from build123d import *

# Parameters (mm, degrees)
F0_R        = 15.113
F0_R_2      = 2.0114491118
F1_DEPTH    = 2.54
F2_T1_DEPTH = 2.54
F2_T3_DEPTH = 27.94


# Not quite as in the source:
# - a fillet or chamfer that OpenCascade refuses, or shapes differently, is made with other operations: its cross-section is extruded or revolved along the edge and cut away or added


with BuildPart() as f1:
    # F0 (on Top) → F1 (new body)
    with BuildSketch(Plane.XY):
        with BuildLine():
            Line((27.3455847055, 4.693207435), (17.2810431679, 4.693207435))
            ThreePointArc((17.2810431679, 4.693207435), (-17.907, 0), (17.2810431679, -4.693207435))
            Line((17.2810431679, -4.693207435), (27.3455847055, -4.693207435))
            Line((27.3455847055, -4.693207435), (27.3455847055, 4.693207435))
        make_face()
        Circle(F0_R, mode=Mode.SUBTRACT)
        with Locations((22.3272647709, 0)):
            Circle(F0_R_2, mode=Mode.SUBTRACT)
    extrude(amount=F1_DEPTH)

    # F2: fillet of radius 5.08 on 4 edges, made by hand

    # F2_s2 → F2_t1 (join)
    with BuildSketch(Plane.XY):
        with BuildLine():
            ThreePointArc((16.2079318414, 7.6133825875), (18.0824647595, 5.4849496171), (20.8059266901, 4.693207435))
            Line((20.8059266901, 4.693207435), (17.2810431679, 4.693207435))
            ThreePointArc((17.2810431679, 4.693207435), (16.8080253904, 6.1766440301), (16.2079318414, 7.6133825875))
        make_face()
        with BuildLine():
            ThreePointArc((16.2079318414, -7.6133825875), (18.0824647595, -5.4849496171), (20.8059266901, -4.693207435))
            Line((20.8059266901, -4.693207435), (17.2810431679, -4.693207435))
            ThreePointArc((17.2810431679, -4.693207435), (16.8080253904, -6.1766440301), (16.2079318414, -7.6133825875))
        make_face()
    extrude(amount=F2_T1_DEPTH)

    # F2_s4 → F2_t3 (cut)
    with BuildSketch(Plane.XY.offset(-12.7)):
        with BuildLine():
            ThreePointArc((22.2655847055, -4.693207435), (25.8576871539, -3.2053098834), (27.3455847055, 0.386792565))
            Line((27.3455847055, 0.386792565), (27.3455847055, -4.693207435))
            Line((27.3455847055, -4.693207435), (22.2655847055, -4.693207435))
        make_face()
        with BuildLine():
            ThreePointArc((27.3455847055, -0.386792565), (25.8576871539, 3.2053098834), (22.2655847055, 4.693207435))
            Line((22.2655847055, 4.693207435), (27.3455847055, 4.693207435))
            Line((27.3455847055, 4.693207435), (27.3455847055, -0.386792565))
        make_face()
    extrude(amount=F2_T3_DEPTH, mode=Mode.SUBTRACT)


solid = f1.part
Geometry check sheet. Reference: the model listing, model coordinates, mm. A direction names the side the tool comes from. Give positions to 0.01 mm unless a question says otherwise; leave off trailing zeros. Write each loop counter-clockwise with the first axis right and the second up, starting at its lowest first coordinate (ties: lowest second). Pieces come first, ordered by that corner, then holes. Notation, with made-up numbers: (-37.75, -20) - (-18.75, -20) arc R20 cw to (-18.75, 14) - close; hole circle Ø1 at (-34.75, -10.5). An arc over 180 degrees is marked (long way). Put each result on its own line as item: value.
1. Sectioned sample at B-B, the plane x = 0. Enter the section's corners in (y, z).
Ans:
outline: (-17.91, 0) - (-15.11, 0) - (-15.11, 2.54) - (-17.91, 2.54) - close; (15.11, 0) - (17.91, 0) - (17.91, 2.54) - (15.11, 2.54) - close
2. Draft check along Y on faces 1 (the cylindrical face through (-17.894, 0.677, 1.252)), 2 (the cylindrical face through (18.049, 5.507, 1.252)), 3 (the cylindrical face through (18.049, -5.507, 1.252)), 4 (the cylindrical face through (-11.14, 10.21, 1.25)). Enter one of: +Y half, -Y half, draft (parallel to the pull), parting line (faces both ways), or undercut.
Ans:
face 1: parting line
face 2: +Y half
face 3: -Y half
face 4: undercut
3. Set-up check for faces 5 (the flat face through (22, -4.693, 1)), 6 (the flat face through (22, 4.693, 1)), 7 (the flat face through (15, 3, 2.54)): record each of +Z, -Z, +X, -X, +Y, -Y from which the full face is reachable in a straight line by a thin tool's end or side.
Ans:
face 5: +Z, -Z, +X, -Y
face 6: +Z, -Z, +X, +Y
face 7: +Z, +X, -X, +Y, -Y
4. Thickness scan on line 1 (Y direction, x = 0, z = 1.5); line 2 (Y direction, x = 5.5, z = 2.4); line 3 (X direction, y = 12.5, z = 0.6). Record the ranges inside material, lowest first.
Ans:
line 1: y = -17.91 to -15.11, 15.11 to 17.91
line 2: y = -17.04 to -14.08, 14.08 to 17.04
line 3: x = -12.82 to -8.49, 8.49 to 12.82
5. Sectioned sample at A-A, the plane z = 1.15. Enter the section's corners in (x, y), plus the area to 3 significant figures.
Ans:
outline: (16.21, -7.61) arc R5.08 cw to (20.81, -4.69) - (22.27, -4.69) arc R5.08 ccw to (27.33, 0) arc R5.08 ccw to (22.27, 4.69) - (20.81, 4.69) arc R5.08 cw to (16.21, 7.61) arc R17.91 ccw (long way) to start; hole circle Ø30.23 at (0, 0); hole circle Ø4.02 at (22.33, 0)
area: 361 mm²
6. Go/stop test with flat-tipped pins: pin 1 (8 mm diameter, centred on x = -9, y = -2, fed in from +Z); pin 2 (1 mm diameter, centred on y = -1.5, z = 0.5, fed in from -X). Record where each tip stops, or that it passes through.
Ans:
pin 1: passes through
pin 2: stops at x = -17.88
7. Sectioned sample at C-C, the plane y = 10. Enter the section's corners in (x, z), plus the area to 3 significant figures.
Ans:
outline: (-14.85, 0) - (-11.33, 0) - (-11.33, 2.54) - (-14.85, 2.54) - close; (11.33, 0) - (14.85, 0) - (14.85, 2.54) - (11.33, 2.54) - close
area: 17.9 mm²
